Work out the finished part from the listing and answer in its coordinate system (mm). A direction names the side the tool comes from. Coordinates: 2 decimals unless noted, no trailing zeros. Write each loop counter-clockwise with the first axis right and the second up, starting at its lowest first coordinate (ties: lowest second). Pieces come first, ordered by that corner, then holes. Notation, with made-up numbers: (23.5, 7) - (58.5, 7) arc R14 ccw to (58.5, 24) - close; hole circle Ø3 at (13.5, 13.5). An arc over 180 degrees is marked (long way). Use one line per item in the form item = value. Start each with the question number.
Item 1: A cutting plane is placed at B-B (z = 46). Write down the section's boundary in (x, y).
Item 2: A cutting plane is placed at A-A (x = -3). Write down the section's boundary in (y, z), then the cut area to 3 significant figures.
Item 3: Given pin 1 (9 mm diameter, centred on y = -11, z = 47, fed in from +X); pin 2 (12 mm diameter, centred on y = -15, z = 4, fed in from +X); pin 3 (4 mm diameter, centred on x = 35, z = 35.5, fed in from -Y); pin 4 (4.5 mm diameter, centred on x = -26.5, y = -17.5, fed in from -Z), each flat-ended and moving along its own axis, determine where each tip first touches the part or whether it passes through.
Item 4: Determine the mould class of faces 1 (the flat face through (-5, -2.6, 15.9)), 2 (the flat face through (13.11, -13, 0)), 3 (the flat face through (44.364, -12.593, 20.699)) for opening direction Z: released by +Z, released by -Z, zero draft, split by the parting line, or undercut.
Item 5: For faces 4 (the cylindrical face through (-32, -22.55, -16.93)), 5 (the cylindrical face through (9.02, -1.53, -16.93)), 6 (the flat face through (8, -13, -18.379)), determine the directions among +Z, -Z, +X, -X, +Y, -Y from which every point of the face is accessible in a straight line to the end or side of a thin tool.
Item 6: A cutting plane is placed at C-C (y = -11.25). Write down the section's boundary in (x, z), then the cut area to 3 significant figures.
Item 7: Consider probe 1 along Z at (x, y) = (-11, -18); probe 2 along Z at (x, y) = (-7, -9.25); probe 3 along Z at (x, y) = (-8, -9.5). Determine where each line is inside the solid, lowest interval first.
Item 8: A cutting plane is placed at D-D (z = -32.5). Write down the section's boundary in (x, y), then the cut area to 3 significant figures.
from build123d import *

# Parameters (mm, degrees)
F0_R     = 4.998133971
F1_DEPTH = 25.4
F2_R     = 5.08
F3_SIZE  = 5.08
F4_SIZE  = 5.08
F5_R     = 5.08
F6_R     = 5.08
F7_R     = 5.08
F8_R     = 5.08
F9_R     = 5.08


with BuildPart() as f1:
    # F0 (on Front) → F1 (new body)
    with BuildSketch(Plane.XZ):
        Polygon((-13.9009580016, -18.3790195733), (36.3904610276, -18.3790195733), (36.3904610276, 11.5175191313), (36.3904610276, 18.3790195733), (21.9322983176, 18.3790195733), (-36.3904610276, 18.3790195733), (-36.3904610276, -18.3790195733), (-22.7228868753, -18.3790195733), (-22.7228868753, -41.6591130197), (0, -41.6591130197), (0, -34.5525592566), (-13.9009580016, -34.5525592566), align=None)
        Polygon((-8.2092965022, 0), (13.1103685126, 9.0669831261), (13.1103685126, -9.5570906997), align=None, mode=Mode.SUBTRACT)
        Polygon((36.3904610276, 18.3790195733), (36.3904610276, 11.5175191313), (52.5639988482, 30.1415920258), (78.7847340107, 30.1415920258), (78.7847340107, 43.3744862676), (78.7847340107, 56.6073805094), (40.0662571192, 56.6073805094), (40.0662571192, 37.4673998365), (21.9322983176, 18.3790195733), align=None)
        with Locations((69.7177499533, 49.2557734251)):
            Circle(F0_R, mode=Mode.SUBTRACT)
        Polygon((78.7847340107, 43.3744862676), (78.7847340107, 30.1415920258), (97.1637517214, 34.7976125777), align=None)
    extrude(amount=F1_DEPTH)

    # F2
    f2_edges = [f1.edges().sort_by_distance(p)[0] for p in [
        (0, -12.7, -34.552559),
    ]]
    fillet(f2_edges, radius=F2_R)

    # F3
    f3_edges = [f1.edges().sort_by_distance(p)[0] for p in [
        (-7.229081, -25.4, 18.37902),
        (-36.390461, -25.4, 0),
    ]]
    chamfer(f3_edges, length=F3_SIZE)

    # F4
    f4_edges = [f1.edges().sort_by_distance(p)[0] for p in [
        (-7.229081, 0, 18.37902),
        (-36.390461, 0, 0),
    ]]
    chamfer(f4_edges, length=F4_SIZE)

    # F5
    f5_edges = [f1.edges().sort_by_distance(p)[0] for p in [
        (-36.390461, -12.7, 18.37902),
    ]]
    fillet(f5_edges, radius=F5_R)

    # F6
    f6_edges = [f1.edges().sort_by_distance(p)[0] for p in [
        (78.784734, -12.7, 56.607381),
        (40.066257, -12.7, 56.607381),
    ]]
    fillet(f6_edges, radius=F6_R)

    # F7
    f7_edges = [f1.edges().sort_by_distance(p)[0] for p in [
        (36.390461, -12.7, -18.37902),
    ]]
    fillet(f7_edges, radius=F7_R)

    # F8
    f8_edges = [f1.edges().sort_by_distance(p)[0] for p in [
        (-36.390461, -12.7, -18.37902),
        (-33.850461, -22.86, -18.37902),
        (-33.850461, -2.54, -18.37902),
    ]]
    fillet(f8_edges, radius=F8_R)

    # F9
    f9_edges = [f1.edges().sort_by_distance(p)[0] for p in [
        (30.999278, -25.4, 27.92321),
        (30.999278, 0, 27.92321),
        (44.47723, -25.4, 20.829556),
        (36.390461, -25.4, -0.89075),
        (44.47723, 0, 20.829556),
        (36.390461, 0, -0.89075),
    ]]
    fillet(f9_edges, radius=F9_R)


solid = f1.part
Answer:
q1.outline = (40.07, -25.4) - (65.93, -25.4) - (65.93, 0) - (40.07, 0) - close; (73.51, -25.4) - (78.78, -25.4) - (78.78, 0) - (73.51, 0) - close
q2.outline = (-25.4, -41.66) - (0, -41.66) - (0, -35) - (-25.4, -35) - close; (-25.4, -13.3) arc R5.08 ccw to (-20.32, -18.38) - (-5.08, -18.38) arc R5.08 ccw to (0, -13.3) - (0, -2.34) - (-25.4, -2.34) - close; (-25.4, 2.22) - (0, 2.22) - (0, 13.3) - (-5.08, 18.38) - (-20.32, 18.38) - (-25.4, 13.3) - close
q2.area = 950 mm²
q3.pin_1 = 80.66
q3.pin_2 = 36.39
q3.pin_3 = through
q3.pin_4 = -18.38
q4.face_1 = released by +Z
q4.face_2 = undercut
q4.face_3 = released by -Z
q5.face_4 = -Z, -X, -Y
q5.face_5 = +X, +Y
q5.face_6 = +X, +Y, -Y
q6.outline = (-36.39, -13.3) arc R5.08 ccw to (-31.31, -18.38) - (-22.72, -18.38) - (-22.72, -41.66) - (0, -41.66) - (0, -39.63) arc R5.08 ccw to (-5.08, -34.55) - (-13.9, -34.55) - (-13.9, -18.38) - (31.31, -18.38) arc R5.08 ccw to (36.39, -13.3) - (36.39, 11.52) - (52.56, 30.14) - (78.78, 30.14) - (97.16, 34.8) - (78.78, 43.37) - (78.78, 51.53) arc R5.08 ccw to (73.7, 56.61) - (45.15, 56.61) arc R5.08 ccw to (40.07, 51.53) - (40.07, 37.47) - (21.93, 18.38) - (-31.31, 18.38) arc R5.08 ccw to (-36.39, 13.3) - close; hole (-8.21, 0) - (13.11, -9.56) - (13.11, 9.07) - close; hole circle Ø10 at (69.72, 49.26)
q6.area = 4,100 mm²
q7.probe_1 = -41.66 to -34.55, -18.38 to 18.38
q7.probe_2 = -41.66 to -34.55, -18.38 to -0.54, 0.51 to 18.38
q7.probe_3 = -41.66 to -34.55, -18.38 to -0.09, 0.09 to 18.38
q8.outline = (-22.72, -25.4) - (-13.9, -25.4) - (-13.9, 0) - (-22.72, 0) - close
q8.area = 224 mm²
